Can you work these out from the model? Positions are in its coordinate system, mm. A direction names the side the tool comes from. Coordinates: 2 decimals unless noted, no trailing zeros. Write each loop counter-clockwise with the first axis right and the second up, starting at its lowest first coordinate (ties: lowest second). Pieces come first, ordered by that corner, then holes. Notation, with made-up numbers: M -32.5,25.25 L -6.5,25.25 A14 cw -6.5,30.25 Z; hole C 85,-25.5 d11. An arc over 180 degrees is marked long. Answer as a JSON object with one key per item and string values. Group by question number.
Autodesk Inventor part; units mm, degrees
ref_plane "YZ Plane" through (0, 0, 0) normal (1, 0, 0) x (0, 1, 0)
ref_plane "XZ Plane" through (0, 0, 0) normal (0, 1, 0) x (-1, 0, 0)
ref_plane "XY Plane" through (0, 0, 0) normal (0, 0, 1) x (1, 0, 0)
sketch "Sketch1" plane through (0, 0, 0) normal (0, 0, 1) x (1, 0, 0)
  circle A0 centre (0, 0) radius 24
  circle A1 centre (0, 0) radius 7.55
  dimension "d0" = 48
  dimension "d1" = 15.1
extrude "Extrusion1" add sketch "Sketch1" along normal blind 3.18
sketch "Sketch2" plane through (0, 0, 0) normal (0, 0, -1) x (-1, 0, 0)
  circle A0 centre (-16.5319, -11.256) radius 2.05
  circle A1 centre (-19.649, 3.7306) radius 2.05
  circle A2 centre (-17.0544, -2.5903) radius 1.65
  circle A3 centre (-6.284, -16.0647) radius 1.65
  circle A4 centre (-6.284, -16.0647) radius 1.65
  circle A5 centre (0, 0) radius 7.55
  line L0 (0, 0) -> (0, -29.2074)
  line L1 (0, 0) -> (-14.8823, -25.7769)
  circle A6 centre (0, 0) radius 17.25
  circle A7 centre (-8.625, -14.9389) radius 2.05
  circle A8 centre (8.625, -14.9389) radius 2.05
  circle A9 centre (17.25, 0) radius 2.05
  circle A10 centre (8.625, 14.9389) radius 2.05
  circle A11 centre (-8.625, 14.9389) radius 2.05
  circle A12 centre (-17.25, 0) radius 2.05
  dimension "d26" = 30
  dimension "d27" = 4.1
  dimension "d30" = 360
extrude "Extrusion2" cut sketch "Sketch2" against normal through all contours A12 A6 A2 | A2 A6 A12 | A6 A12 A2 | A2 A12 A6 | A7 L1 A6 | A6 L1 A7 | A6 A3 A7 L1 | L1 A7 A3 A6 | A11 A6 | A6 A11 | A6 A7 A3 | A3 A7 A6 | A10 A6 | A6 A10 | A8 A6 | A6 A8 | A9 A6 | A6 A9 picked at (-16.7628, -1.5642) picked at (-16.3049, -0.3328) picked at (-17.5539, -1.6273) picked at (-18.131, -0.5464) picked at (-7.3677, -16.0157) picked at (-7.0171, -15.2489)
sketch "Sketch3" plane through (0, 0, 3.18) normal (0, 0, 1) x (1, 0, 0)
  line L0 (-2.5, 4.5) -> (-2.5, 7.0711)
  arc A0 (-2.5, 7.0711) -> (2.5, 7.0711) centre (0, 0) ccw
  line L1 (2.5, 7.0711) -> (2.5, 4.5)
  line L2 (2.5, 4.5) -> (-2.5, 4.5)
  line L3 (-2.4503, 4.5542) -> (2.4493, 4.5542)
  line L4 (2.4493, 4.5542) -> (2.4493, 8.0911)
  line L5 (2.4493, 8.0911) -> (-2.4503, 8.0911)
  line L6 (-2.4503, 8.0911) -> (-2.4503, 4.5542)
  circle A1 centre (0, 0) radius 7.55
  dimension "d16" = 7.5
  dimension "d17" = 5
  dimension "d18" = 2.9958
extrude "Extrusion3" add sketch "Sketch3" against normal up to surface (3.18 mm away) contours L6 A1 L4 L3 | L6 L5 L4 A1 picked at (-0.2772, 5.5375)
chamfer "Chamfer1" distance 0.2 angle 45 2 edges at (-2.4503, 4.5542, 1.59) (2.4493, 4.5542, 1.59)
properties part number "spool_spacer_driver"
Q1. We'd pull the mould along X, two halves only. Please class faces 3 (the flat face through (0, 6, 3.18)), 4 (the cylindrical face through (-23.977, -1.055, 1.568)), 5 (the cylindrical face through (-15.2, 0.09, 1.57)): pulls with the +X half, pulls with the -X half, needs draft (parallel to the pull), parting line crosses it, or undercut.
Q2. On a 3-axis mill with a long thin cutter (end or side, diameter ignored), from which of +Z, -Z, +X, -X, +Y, -Y can I reach the whole of each face in a straight line? I mean faces 1 (the flat face through (-2.45, 6, 2)), 2 (the flat face through (0, 6, 0)). Say none if no direction works.
Q3. Will these pins go through, and if not, where does the flat tip stop? pin 1 (2 mm diameter, centred on x = 2.5, y = -13.5, fed in from -Z); pin 2 (1.2 mm diameter, centred on y = 6, z = 2.5, fed in from -X); pin 3 (1 mm diameter, centred on x = -0.5, z = 1, fed in from -Y); pin 4 (1 mm diameter, centred on y = -13, z = 0.5, fed in from +X).
Q4. If we section it at B-B on y = 0: List the corners of the cut face in (x, z) for me.
Q5. If we section it at D-D on y = -7: List the corners of the cut face in (x, z) for me.
Q6. If we section it at A-A on x = 0: List the corners of the cut face in (y, z) for me.
Q7. Please list where these lines run through material, in increasing order: L1, parallel to Y at x = 7, z = 1.3; L2, parallel to Y at x = 9, z = 1.6; L3, parallel to X at y = -1.5, z = 1.6.
Q8. If we section it at C-C on z = 1.85: List the corners of the cut face in (x, y) for me (3 decimals), and give its area (3 significant figures).
Reply:
{
 "1": {"face 3": "needs draft", "face 4": "parting line crosses it", "face 5": "undercut"},
 "2": {"face 1": "+Z, -Z", "face 2": "-Z, +X, -X, +Y, -Y"},
 "3": {"pin 1": "z = 0", "pin 2": "x = -23.38", "pin 3": "y = -24", "pin 4": "x = 20.49"},
 "4": {"outline": "M -24,0 L -19.3,0 L -19.3,3.18 L -24,3.18 Z; M -15.2,0 L -7.55,0 L -7.55,3.18 L -15.2,3.18 Z; M 7.55,0 L 15.2,0 L 15.2,3.18 L 7.55,3.18 Z; M 19.3,0 L 24,0 L 24,3.18 L 19.3,3.18 Z"},
 "5": {"outline": "M -22.96,0 L -2.83,0 L -2.83,3.18 L -22.96,3.18 Z; M 2.83,0 L 22.96,0 L 22.96,3.18 L 2.83,3.18 Z"},
 "6": {"outline": "M -24,0 L -7.55,0 L -7.55,3.18 L -24,3.18 Z; M 4.55,0 L 24,0 L 24,3.18 L 4.55,3.18 Z"},
 "7": {"L1": "-22.96 to -16.19, -13.69 to -2.83, 2.83 to 13.69, 16.19 to 22.96", "L2": "-22.25 to -16.95, -12.92 to 12.92, 16.95 to 22.25", "L3": "-23.95 to -18.65, -15.85 to -7.4, 7.4 to 15.85, 18.65 to 23.95"},
 "8": {"outline": "C 0,0 d48; hole C -17.25,0 d4.1; hole C -8.625,-14.939 d4.1; hole C -8.625,14.939 d4.1; hole M -2.45,4.754 L -2.45,7.141 A7.55 ccw long 2.449,7.142 L 2.449,4.754 L 2.249,4.554 L -2.25,4.554 Z; hole C 8.625,-14.939 d4.1; hole C 8.625,14.939 d4.1; hole C 17.25,0 d4.1", "area": "1,570 mm^2"}
}
